Geometry: final body of the model. Coordinates: model frame, mm. Give positions to 0.01 mm unless a question says otherwise; leave off trailing zeros. Write each loop counter-clockwise with the first axis right and the second up, starting at its lowest first coordinate (ties: lowest second). Pieces come first, ordered by that corner, then holes. Notation, with made-up numbers: (16, 56.5) -> (70, 56.5) arc R32 cw to (70, 84.5) -> close; hole circle Ø2 at (62.25, -22.75). An arc over 180 degrees is marked (long way). Answer in a Markdown table with one row per item. Add a question column.
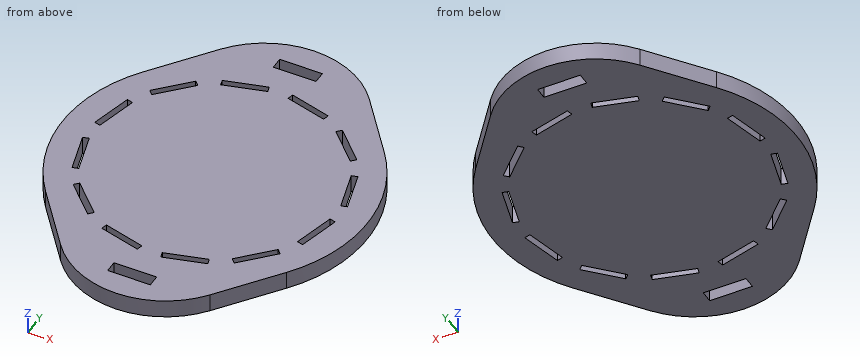
from build123d import *

# Parameters (mm, degrees)
PAD_DEPTH             = 1.5
SKETCH006_W           = 3.5
SKETCH006_H           = 1
POCKET_DEPTH          = 81.206709
POLARPATTERN_COUNT    = 2
SKETCH014_W           = 0.5
SKETCH014_H           = 3.5
POCKET004_DEPTH       = 81.206709
POLARPATTERN003_COUNT = 12


with BuildPart() as part:
    # Sketch → Pad (new body)
    with BuildSketch(Plane.XY):
        with BuildLine():
            ThreePointArc((-9.876975, 7.66129), (-12.5, 0), (-9.876975, -7.66129))
            Line((-9.876975, -7.66129), (-6.123724, -12.5))
            ThreePointArc((-6.123724, -12.5), (0, -15.5), (6.123724, -12.5))
            Line((6.123724, -12.5), (9.876996, -7.661263))
            ThreePointArc((9.876996, -7.661263), (12.5, 0), (9.876996, 7.661263))
            Line((6.123742, 12.499977), (9.876996, 7.661263))
            ThreePointArc((6.123742, 12.499977), (1.7e-05, 15.5), (-6.123722, 12.500003))
            Line((-9.876975, 7.66129), (-6.123722, 12.500003))
        make_face()
    extrude(amount=PAD_DEPTH)

    # Sketch006 → Pocket (cut, through all)
    with BuildSketch(Plane.XY):
        with Locations((0, -13)):
            Rectangle(SKETCH006_W, SKETCH006_H)
    pocket = extrude(amount=POCKET_DEPTH, mode=Mode.SUBTRACT)

    # PolarPattern: Pocket ×2 about axis
    polarpattern_axis = Axis((0, 0, 0), (0, 0, 1))
    for i in range(1, POLARPATTERN_COUNT):
        add(pocket.rotate(polarpattern_axis, i * 360 / POLARPATTERN_COUNT), mode=Mode.SUBTRACT)

    # Sketch014 → Pocket004 (cut, through all)
    with BuildSketch(Plane(origin=(0, 0, 0), x_dir=(0.965926, 0.258819, 0), z_dir=(0, 0, 1))):
        with Locations((-10, 0)):
            Rectangle(SKETCH014_W, SKETCH014_H)
    pocket004 = extrude(amount=POCKET004_DEPTH, mode=Mode.SUBTRACT)

    # PolarPattern003: Pocket004 ×12 about axis
    polarpattern003_axis = Axis((0, 0, 0), (0, 0, 1))
    for i in range(1, POLARPATTERN003_COUNT):
        add(pocket004.rotate(polarpattern003_axis, i * 360 / POLARPATTERN003_COUNT), mode=Mode.SUBTRACT)


solid = part.part
Q1. Line query: probe 1 along X at (y, z) = (7, 0.3); probe 2 along Y at (x, z) = (2.5, 0.45); probe 3 along Y at (x, z) = (3.5, 0.5). Output: solid intervals per line, ascending. Write a range as from..to.
Q2. Section D-D on z = 0.3. Count the separate pieces of the cut face and the enclosed holes in it, and give its area (3 significant figures).
Q3. Contact query for a flat-ended pin moving along its axis: pin 1 Ø0.8 at (y, z) = (13, 0.5) entering from +X. Output: stop coordinate, or through.
Q4. Section B-B on x = 2.75. Return loops of the section in (y, z), and give its area (3 significant figures).
Q5. Section A-A on y = -13. Return loops of the section in (x, z), and give its area (3 significant figures).
Q6. Section C-C on y = 6.5. Return loops of the section in (x, z).
Checks:
| question | item | result |
|---|---|---|
| 1 | probe 1 | -10.36..-7.5, -6.79..6.79, 7.5..10.36 |
| 1 | probe 2 | -15.09..-9.94, -9.42..9.42, 9.94..15.09 |
| 1 | probe 3 | -14.66..-9.67, -9.16..9.16, 9.67..14.66 |
| 2 | separate pieces | 1 |
| 2 | enclosed holes | 14 |
| 2 | area | 536 mm^2 |
| 3 | pin 1 | x = 6.04 |
| 4 | outline | (-15, 0) -> (-9.87, 0) -> (-9.87, 1.5) -> (-15, 1.5) -> close; (-9.36, 0) -> (9.36, 0) -> (9.36, 1.5) -> (-9.36, 1.5) -> close; (9.87, 0) -> (15, 0) -> (15, 1.5) -> (9.87, 1.5) -> close |
| 4 | area | 43.4 mm^2 |
| 5 | outline | (-5.7, 0) -> (-1.75, 0) -> (-1.75, 1.5) -> (-5.7, 1.5) -> close; (1.75, 0) -> (5.7, 0) -> (5.7, 1.5) -> (1.75, 1.5) -> close |
| 5 | area | 11.9 mm^2 |
| 6 | outline | (-10.68, 0) -> (-8, 0) -> (-8, 1.5) -> (-10.68, 1.5) -> close; (-7.29, 0) -> (7.29, 0) -> (7.29, 1.5) -> (-7.29, 1.5) -> close; (8, 0) -> (10.68, 0) -> (10.68, 1.5) -> (8, 1.5) -> close |
